For this review, take the finished solid that the model builds, in its own axes (mm). Face numbers are marked on the shaded views. A direction names the side the tool comes from. Round coordinates to 2 decimals unless told otherwise and drop trailing zeros. Write each loop counter-clockwise with the first axis right and the second up, starting at its lowest first coordinate (ties: lowest second). Pieces come first, ordered by that corner, then holes. Notation, with made-up numbers: (-15.75, 83) -> (-9.75, 83) arc R25 ccw to (-9.75, 113) -> close; hole circle Ø10 at (29.5, 33.25). An arc over 180 degrees is marked (long way). Answer in a Markdown table with one row per item.
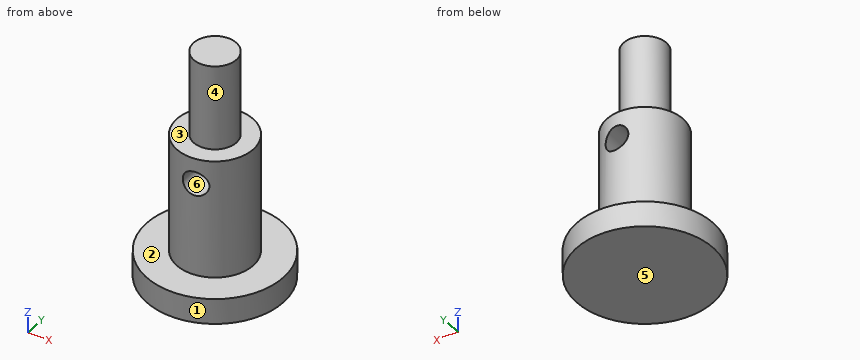
from build123d import *

# Parameters (mm, degrees)
SKETCH1_R           = 8
BOSS_EXTRUDE1_DEPTH = 3
SKETCH2_R           = 4.475
BOSS_EXTRUDE2_DEPTH = 14
SKETCH3_R           = 2.5
BOSS_EXTRUDE3_DEPTH = 10
SKETCH4_R           = 1.425
CUT_EXTRUDE1_DEPTH  = 7.5


with BuildPart() as part:
    # Sketch1 → Boss-Extrude1 (new body)
    with BuildSketch(Plane.XY):
        Circle(SKETCH1_R)
    extrude(amount=BOSS_EXTRUDE1_DEPTH)

    # Sketch2 → Boss-Extrude2 (add)
    with BuildSketch(Plane.XY.offset(3)):
        Circle(SKETCH2_R)
    extrude(amount=BOSS_EXTRUDE2_DEPTH)

    # Sketch3 → Boss-Extrude3 (add)
    with BuildSketch(Plane.XY.offset(17)):
        Circle(SKETCH3_R)
    extrude(amount=BOSS_EXTRUDE3_DEPTH)

    # Sketch4 → Cut-Extrude1 (cut, symmetric)
    with BuildSketch(Plane(origin=(0, 0, 0), x_dir=(1, 0, 0), z_dir=(0, 1, 0))):
        with Locations((0.525, -13.990152787)):
            Circle(SKETCH4_R)
    extrude(amount=CUT_EXTRUDE1_DEPTH, both=True, mode=Mode.SUBTRACT)


solid = part.part
1) For the marked faces 1 and 2, list the 3-axis set-ups (+Z, -Z, +X, -X, +Y, -Y) from which the entire face can be reached by the end or side of a thin tool; tool diameter is ignored.
Solved:
| item | result |
|---|---|
| face 1 | +Z, -Z |
| face 2 | +Z |
2) Clearance check with flat-ended pins moving along their axes: pin 1 Ø1.5 at (x, y) = (-3, 3) entering from +Z; pin 2 Ø1 at (y, z) = (-4.5, 13) entering from +X; pin 3 Ø4.5 at (x, z) = (0.52, 13.99) entering from +Y (3 decimals). State where each tip first meets the part, or that it passes through.
Solved:
| item | result |
|---|---|
| pin 1 | z = 17 |
| pin 2 | x = 2.01 |
| pin 3 | y = 4.475 |
3) Mouldability with a two-part tool opening along Z and no side actions: class the marked faces 3, 4, 5 and 6 as pulls with the +Z half, pulls with the -Z half, needs draft (parallel to the pull), parting line crosses it, or undercut.
Solved:
| item | result |
|---|---|
| face 3 | pulls with the +Z half |
| face 4 | needs draft |
| face 5 | pulls with the -Z half |
| face 6 | undercut |
4) For line 1 (Z direction, x = 5, y = -2.25); line 2 (Z direction, x = 1.5, y = -3.5); line 3 (Z direction, x = -0.25, y = -3), list the stretches that pass through material, from the lowest coordinate up. Write a range as [from, to].
Solved:
| item | result |
|---|---|
| line 1 | [0, 3] |
| line 2 | [0, 12.95], [15.03, 17] |
| line 3 | [0, 12.79], [15.19, 17] |
5) Consider section D-D on x = 3. State the section outline as (y, z) points, then the cut area to 3 significant figures.
Solved:
| item | result |
|---|---|
| outline | (-7.42, 0) -> (7.42, 0) -> (7.42, 3) -> (3.32, 3) -> (3.32, 17) -> (-3.32, 17) -> (-3.32, 3) -> (-7.42, 3) -> close |
| area | 137 mm² |
6) Consider section A-A on x = 1. State the section outline as (y, z) points.
Solved:
| item | result |
|---|---|
| outline | (-7.94, 0) -> (7.94, 0) -> (7.94, 3) -> (4.36, 3) -> (4.36, 12.65) -> (-4.36, 12.65) -> (-4.36, 3) -> (-7.94, 3) -> close; (-4.36, 15.33) -> (4.36, 15.33) -> (4.36, 17) -> (2.29, 17) -> (2.29, 27) -> (-2.29, 27) -> (-2.29, 17) -> (-4.36, 17) -> close |
7) Consider section C-C on z = 23.25. State the section outline as (x, y) points, then the cut area to 3 significant figures.
Solved:
| item | result |
|---|---|
| outline | circle Ø5 at (0, 0) |
| area | 19.6 mm² |
8) Consider section B-B on y = 0. State the section outline as (x, z) points (3 decimals), then the cut area to 3 significant figures.
Solved:
| item | result |
|---|---|
| outline | (-8, 0) -> (8, 0) -> (8, 3) -> (4.475, 3) -> (4.475, 17) -> (2.5, 17) -> (2.5, 27) -> (-2.5, 27) -> (-2.5, 17) -> (-4.475, 17) -> (-4.475, 3) -> (-8, 3) -> close; hole circle Ø2.85 at (0.525, 13.99) |
| area | 217 mm² |
